from build123d import *

# Parameters (mm, degrees)
SKETCH1_R           = 4
BOSS_EXTRUDE1_DEPTH = 129.988767867
SKETCH3_R           = 2
CUT_EXTRUDE1_DEPTH  = 19.5


with BuildPart() as part:
    # Sketch1 → Boss-Extrude1 (new body)
    with BuildSketch(Plane(origin=(0, 0, 0), x_dir=(1, 0, 0), z_dir=(0, 1, 0))):
        with Locations(Location((0, 0, 0), (0, 0, 270))):
            Circle(SKETCH1_R)
    extrude(amount=BOSS_EXTRUDE1_DEPTH)

    # Loft1: read off the stored shape, not the designer's step
    # Loft1: loft between two sections, ruled curve by curve
    loft1_from = [
        Edge.make_bspline([(0, -15, -0.05), (-0.1, -15, -0.05), (-0.1, -15, 0.05), (0, -15, 0.05), (0.1, -15, 0.05), (0.1, -15, -0.05), (0, -15, -0.05)], [0, 0, 0, 0, 0.5, 0.5, 0.5, 1, 1, 1, 1], 3, [1, 0.333333333, 0.333333333, 1, 0.333333333, 0.333333333, 1]),
    ]
    loft1_to = [
        Edge.make_bspline([(3.965560399, 0, 0.523765905), (5.013092209, 0, -7.407354893), (-2.918028589, 0, -8.454886703), (-3.965560399, 0, -0.523765905), (-5.013092209, 0, 7.407354893), (2.918028589, 0, 8.454886703), (3.965560399, 0, 0.523765905)], [0, 0, 0, 0, 0.5, 0.5, 0.5, 1, 1, 1, 1], 3, [1, 0.333333333, 0.333333333, 1, 0.333333333, 0.333333333, 1]),
    ]
    loft1 = Solid(Shell([*[Face.make_surface_from_curves(loft1_from[k], loft1_to[k]) for k in range(1)], Face(Wire(loft1_from)), Face(Wire(loft1_to))]))
    add(loft1)

    # Sketch3 → Cut-Extrude1 (cut, symmetric)
    with BuildSketch(Plane.XY):
        with Locations((0, 120.894404614)):
            Circle(SKETCH3_R)
    extrude(amount=CUT_EXTRUDE1_DEPTH, both=True, mode=Mode.SUBTRACT)


solid = part.part
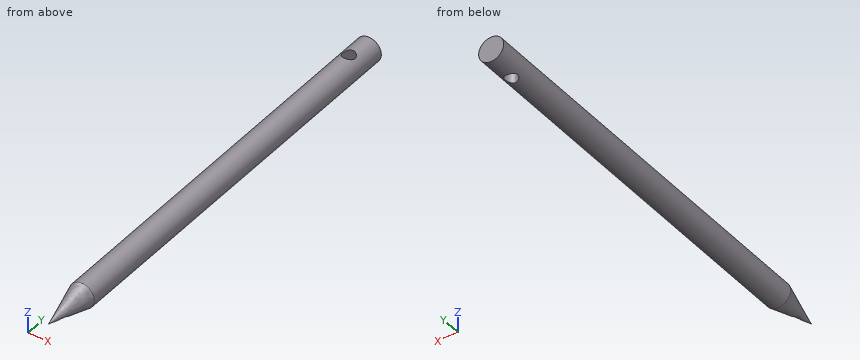
Read the model definition and answer for the solid it produces. Units are mm, in the model's axes. Coordinates: 2 decimals unless noted, no trailing zeros. Order: outer loops, then holes, each group sorted by start corner. A loop starts at its lowest first (then second) coordinate and runs counter-clockwise, first axis right, second up. Notation, with made-up numbers: M -21,-24.5 L 16,-24.5 A27 cw 16,9.5 Z; hole C -16,59 d7. An arc over 180 degrees is marked long. Put each result on its own line as item: value. Start each with the question number.
Item 1: Given pin 1 Ø4 at (y, z) = (8.5, -2.5) entering from +X, flat-ended and moving along its own axis, determine where the tip first touches the part or whether it passes through.
Item 2: Consider probe 1 along X at (y, z) = (120, -2.25); probe 2 along Z at (x, y) = (0.25, 118); probe 3 along X at (y, z) = (120.5, 0.75). Determine where each line is inside the solid, lowest interval first. Write a range as [from, to].
Item 3: Section A-A, the plane y = 81 is taken. Determine the outline of the cut face in (x, z), plus the area to 3 significant figures.
Computed:
1. pin 1: stops at x = 3.97
2. probe 1: x = [-3.31, -1.79], [1.79, 3.31]
2. probe 2: z = [-3.99, 3.99]
2. probe 3: x = [-3.93, -1.96], [1.96, 3.93]
3. outline: C 0,0 d8
3. area: 50.3 mm2
